The listing builds one solid part. Answer for the finished solid, in the listing's coordinates (mm). Coordinates: 2 decimals unless noted, no trailing zeros. Order: outer loops, then holes, each group sorted by start corner. A loop starts at its lowest first (then second) coordinate and runs counter-clockwise, first axis right, second up. Notation, with made-up numbers: M -25,61 L 28,61 A20 cw 28,97 Z; hole C -32.75,31.5 d10. An arc over 180 degrees is marked long. One line per item, written item: value. Start each with the question number.
Q1. The part is cut by section B-B on z = 0.95. Give the number of separate pieces and of enclosed holes in the cut face, then the cut area to 3 significant figures.
Q2. This flat-tipped pin is pushed along its axis until it touches: pin 1 Ø2.5 at (x, y) = (30, -38.5) entering from +Z. Where does it stop, or does it pass through?
Q3. The part is cut by section A-A on x = 0. Give the vertices of the cut face in (y, z), then the cut area to 3 significant figures.
Q4. The part is cut by section D-D on y = 8.75. Give the vertices of the cut face in (x, z), then the cut area to 3 significant figures.
Q5. The part is cut by section C-C on y = 23.5. Give the vertices of the cut face in (x, z).
Q6. Straight lines are drawn through the part: line 1 along X through (y, z) = (-12, 1.4); line 2 along X through (y, z) = (-11, 2.2); line 3 along Y through (x, z) = (-15.5, 0.6). For each, find the intervals that lie inside material, in ascending order. Write a range as [from, to].
```python
from build123d import *

# Parameters (mm, degrees)
SKETCH_1_R          = 13
EXTRUDE_1_DEPTH     = 4
SKETCH_2_R          = 4.5
CUT_EXTRUDE_1_DEPTH = 63.417946137
SKETCH_3_R          = 1.5
CUT_EXTRUDE_5_DEPTH = 4
SKETCH_4_R          = 1.5
CUT_EXTRUDE_6_DEPTH = 63.417946137


with BuildPart() as part:
    # 草图1 → 凸台-拉伸1 (new body)
    with BuildSketch(Plane.XY):
        with BuildLine():
            ThreePointArc((34.64123049, 4.998514795), (0, 35), (-34.64123049, 4.998514795))
            Line((-34.64123049, 4.998514795), (-42, -46))
            Line((-42, -46), (42, -46))
            Line((42, -46), (34.64123049, 4.998514795))
        make_face()
        Circle(SKETCH_1_R, mode=Mode.SUBTRACT)
    extrude(amount=EXTRUDE_1_DEPTH)

    # 草图2 → 切除-拉伸1 (cut, through all)
    with BuildSketch(Plane.XY.offset(4)):
        with Locations((0, 22.5)):
            Circle(SKETCH_2_R)
        with Locations((19.485571585, -11.25)):
            Circle(SKETCH_2_R)
        with Locations((-19.485571585, -11.25)):
            Circle(SKETCH_2_R)
    extrude(amount=-CUT_EXTRUDE_1_DEPTH, mode=Mode.SUBTRACT)

    # 草图3 → 切除-拉伸5 (cut)
    with BuildSketch(Plane.XY):
        with Locations((15.155444566, 8.75)):
            Circle(SKETCH_3_R)
        with Locations((0, -17.5)):
            Circle(SKETCH_3_R)
        with Locations((-15.155444566, 8.75)):
            Circle(SKETCH_3_R)
    extrude(amount=CUT_EXTRUDE_5_DEPTH, mode=Mode.SUBTRACT)

    # 草图4 → 切除-拉伸6 (cut, through all)
    with BuildSketch(Plane.XY.offset(4)):
        with Locations((0, -38.5)):
            Circle(SKETCH_4_R)
        with Locations((-30, -38.5)):
            Circle(SKETCH_4_R)
        with Locations(Location((30, -38.5, 0), (0, 0, 180))):
            Circle(SKETCH_4_R)
    extrude(amount=-CUT_EXTRUDE_6_DEPTH, mode=Mode.SUBTRACT)


solid = part.part
```
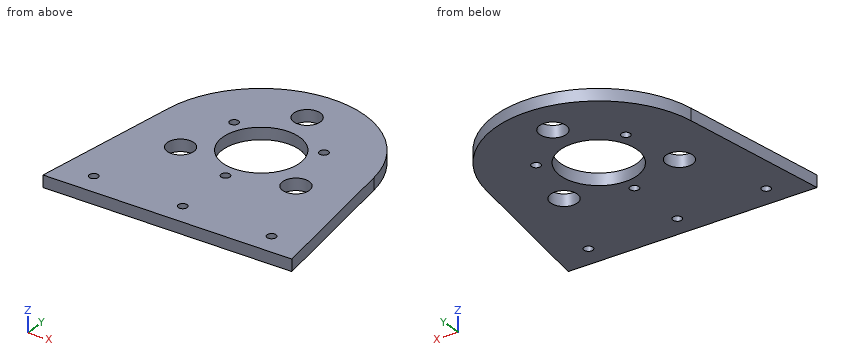
Output:
1. separate pieces: 1
1. enclosed holes: 10
1. area: 4,720 mm^2
2. pin 1: passes through
3. outline: M -46,0 L -40,0 L -40,4 L -46,4 Z; M -37,0 L -19,0 L -19,4 L -37,4 Z; M -16,0 L -13,0 L -13,4 L -16,4 Z; M 13,0 L 18,0 L 18,4 L 13,4 Z; M 27,0 L 35,0 L 35,4 L 27,4 Z
3. area: 160 mm^2
4. outline: M -33.89,0 L -16.66,0 L -16.66,4 L -33.89,4 Z; M -13.66,0 L -9.61,0 L -9.61,4 L -13.66,4 Z; M 9.61,0 L 13.66,0 L 13.66,4 L 9.61,4 Z; M 16.66,0 L 33.89,0 L 33.89,4 L 16.66,4 Z
4. area: 170 mm^2
5. outline: M -25.94,0 L -4.39,0 L -4.39,4 L -25.94,4 Z; M 4.39,0 L 25.94,0 L 25.94,4 L 4.39,4 Z
6. line 1: x = [-37.09, -23.92], [-15.05, -5], [5, 15.05], [23.92, 37.09]
6. line 2: x = [-36.95, -23.98], [-14.99, -6.93], [6.93, 14.99], [23.98, 36.95]
6. line 3: y = [-46, -13.34], [-9.16, 7.29], [10.21, 31.38]
